Design review of the part built by this model. Coordinates are the model's own, in mm. Face numbers are marked on the shaded views. A direction names the side the tool comes from. Give positions to 0.01 mm unless a question says otherwise; leave off trailing zeros. Write each loop counter-clockwise with the first axis right and the second up, starting at its lowest first coordinate (ties: lowest second). Pieces come first, ordered by that corner, then holes.
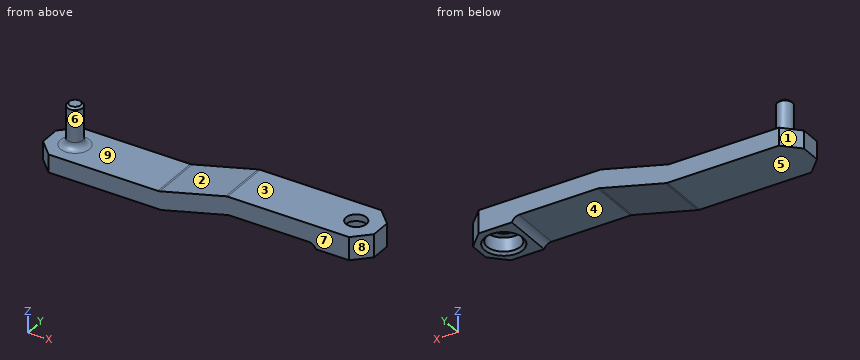
```python
from build123d import *

# Parameters (mm, degrees)
BOSS_EXTRUDE1_DEPTH = 12.7
SKETCH2_R           = 4.1148
CUT_EXTRUDE1_DEPTH  = 4.064
SKETCH3_R           = 2.54
CUT_EXTRUDE2_DEPTH  = 84.509486698
SKETCH4_R           = 1.9304
BOSS_EXTRUDE2_DEPTH = 10.16
FILLET1_R           = 1.651
CHAMFER1_SIZE       = 3.81
FILLET2_R           = 1.905
CHAMFER2_SIZE       = 0.635
CHAMFER3_SIZE       = 0.508


with BuildPart() as part:
    # Sketch1 → Boss-Extrude1 (new body)
    with BuildSketch(Plane(origin=(0, 0, 0), x_dir=(1, 0, 0), z_dir=(0, 1, 0))):
        Polygon((0, 0), (0, -4.445), (31.190740793, -4.445), (48.018240793, -8.7475), (82.2325, -8.7475), (82.2325, -3.0325), (70.1675, -3.0325), (70.1675, -4.3025), (48.5775, -4.3025), (31.75, 0), align=None)
    extrude(amount=BOSS_EXTRUDE1_DEPTH)

    # Sketch2 → Cut-Extrude1 (cut)
    with BuildSketch(Plane(origin=(0, 0, 3.0325), x_dir=(-1, 0, 0), z_dir=(0, 0, -1))):
        with Locations((-76.2, 6.35)):
            Circle(SKETCH2_R)
    extrude(amount=-CUT_EXTRUDE1_DEPTH, mode=Mode.SUBTRACT)

    # Sketch3 → Cut-Extrude2 (cut, through all)
    with BuildSketch(Plane(origin=(0, 0, 7.0965), x_dir=(-1, 0, 0), z_dir=(0, 0, -1))):
        with Locations((-76.2, 6.35)):
            Circle(SKETCH3_R)
    extrude(amount=-CUT_EXTRUDE2_DEPTH, mode=Mode.SUBTRACT)

    # Sketch4 → Boss-Extrude2 (add)
    with BuildSketch(Plane(origin=(0, 0, 4.445), x_dir=(-1, 0, 0), z_dir=(0, 0, -1))):
        with Locations((-6.35, 6.35)):
            Circle(SKETCH4_R)
    extrude(amount=-BOSS_EXTRUDE2_DEPTH)

    # Fillet1
    fillet1_edges = [part.edges().sort_by_distance(p)[0] for p in [
        (8.2804, 6.35, 4.445),
    ]]
    fillet(fillet1_edges, radius=FILLET1_R)

    # Chamfer1
    chamfer1_edges = [part.edges().sort_by_distance(p)[0] for p in [
        (82.2325, 0, 5.89),
        (0, 0, 2.2225),
        (82.2325, 12.7, 5.89),
        (0, 12.7, 2.2225),
    ]]
    chamfer(chamfer1_edges, length=CHAMFER1_SIZE)

    # Fillet2
    # the kernel refuses this fillet: 1.905 mm, written as the material it adds along each edge
    with BuildSketch(Plane(origin=(31.190740793, 0, 4.445), x_dir=(-1, 0, 0), z_dir=(0, 1, 0))) as fillet2_piece_1:
        with BuildLine():
            CenterArc((FILLET2_R * 0.125817594312, FILLET2_R), FILLET2_R, 255.657728572, 14.342271428)
            Line((-FILLET2_R * 0.121896267277, FILLET2_R * 0.0311667621428), (0, 0))
            Line((0, 0), (FILLET2_R * 0.125817594312, 0))
        make_face()
    extrude(amount=12.7)
    with BuildSketch(Plane(origin=(48.5775, 0, 4.3025), x_dir=(-0.96883323785722, 0, -0.24771386158851796), z_dir=(0, 1, 0))) as fillet2_piece_2:
        with BuildLine():
            CenterArc((FILLET2_R * 0.125817594312, -FILLET2_R), FILLET2_R, 90, 14.342271428)
            Line((-FILLET2_R * 0.121896267277, -FILLET2_R * 0.0311667621428), (0, 0))
            Line((0, 0), (FILLET2_R * 0.125817594312, 0))
        make_face()
    extrude(amount=12.7)
    with BuildSketch(Plane(origin=(70.1675, 0, 4.3025), x_dir=(-1, 0, 0), z_dir=(0, 1, 0))) as fillet2_piece_3:
        with BuildLine():
            CenterArc((1.796051224, -1.905), FILLET2_R, 90, 70.528779366)
            Line((0, -1.27), (0, 0))
            Line((0, 0), (1.796051224, 0))
        make_face()
    extrude(amount=12.7)
    # the kernel refuses this fillet: 1.905 mm, written as the material it takes off along each edge
    with BuildSketch(Plane(origin=(48.018240793, -0.599206293, 8.7475), x_dir=(-0.96883323785722, 0, -0.24771386158851796), z_dir=(0, 1, 0))) as fillet2_2_piece_1:
        with BuildLine():
            CenterArc((FILLET2_R * 0.125817594312, -FILLET2_R), FILLET2_R, 90, 14.342271428)
            Line((-FILLET2_R * 0.121896267277, -FILLET2_R * 0.0311667621428), (0, 0))
            Line((0, 0), (FILLET2_R * 0.125817594312, 0))
        make_face()
    extrude(amount=13.898412586, mode=Mode.SUBTRACT)
    with BuildSketch(Plane(origin=(31.75, -0.599206293, 0), x_dir=(-1, 0, 0), z_dir=(0, 1, 0))) as fillet2_2_piece_2:
        with BuildLine():
            CenterArc((FILLET2_R * 0.125817594312, FILLET2_R), FILLET2_R, 255.657728572, 14.342271428)
            Line((-FILLET2_R * 0.121896267277, FILLET2_R * 0.0311667621428), (0, 0))
            Line((0, 0), (FILLET2_R * 0.125817594312, 0))
        make_face()
    extrude(amount=13.898412586, mode=Mode.SUBTRACT)

    # Chamfer2
    chamfer2_edges = [part.edges().sort_by_distance(p)[0] for p in [
        (80.3148, 6.35, 3.0325),
    ]]
    chamfer(chamfer2_edges, length=CHAMFER2_SIZE)

    # Chamfer3
    chamfer3_edges = [part.edges().sort_by_distance(p)[0] for p in [
        (8.2804, 6.35, 14.605),
    ]]
    chamfer(chamfer3_edges, length=CHAMFER3_SIZE)


solid = part.part
```
(1) Mouldability with a two-part tool opening along X and no side actions: class the marked faces 6, 7, 8 and 9 as pulls with the +X half, pulls with the -X half, needs draft (parallel to the pull), parting line crosses it, or undercut.
Resolved:
face 6: undercut
face 7: needs draft
face 8: pulls with the +X half
face 9: undercut
(2) Consider section D-D, the plane z = 2. Give the boundary of the cut face in (x, y).
Resolved:
outline: (0, 3.81) - (3.81, 0) - (39.57, 0) - (39.57, 12.7) - (3.81, 12.7) - (0, 8.89) - close
(3) Tool access review of the marked faces 1, 2, 3, 4 and 5: name each direction out of +Z, -Z, +X, -X, +Y, -Y from which nothing blocks a thin tool from reaching the whole face with its end or side.
Resolved:
face 1: +Z, -Z, -X, +Y
face 2: +Z, +Y, -Y
face 3: +Z, +X, +Y, -Y
face 4: -Z, +Y, -Y
face 5: -Z, +X, -X, +Y, -Y
(4) To check wall thickness, follow L1, parallel to Y at x = 76.2, z = 7.9; L2, parallel to Z at x = 56, y = 5.5; L3, parallel to Z at x = 27.5, y = 9.25 (3 decimals). State the ranges of each line that lie inside material, in increasing order.
Resolved:
L1: y = 0 to 3.81, 8.89 to 12.7
L2: z = 4.3 to 8.75
L3: z = 0 to 4.445
(5) Consider section C-C, the plane x = 6.35. Give the boundary of the cut face in (y, z) (3 decimals).
Resolved:
outline: (0, 0) - (12.7, 0) - (12.7, 4.445) - (9.931, 4.445) arc R1.651 cw to (8.28, 6.096) - (8.28, 14.097) - (7.772, 14.605) - (4.928, 14.605) - (4.42, 14.097) - (4.42, 6.096) arc R1.651 cw to (2.769, 4.445) - (0, 4.445) - close
(6) Consider section A-A, the plane x = 76.2. Give the boundary of the cut face in (y, z), then the cut area to 3 significant figures.
Resolved:
outline: (0, 3.03) - (1.6, 3.03) - (2.24, 3.67) - (2.24, 7.1) - (3.81, 7.1) - (3.81, 8.75) - (0, 8.75) - close; (8.89, 7.1) - (10.46, 7.1) - (10.46, 3.67) - (11.1, 3.03) - (12.7, 3.03) - (12.7, 8.75) - (8.89, 8.75) - close
area: 30.3 mm2
(7) Clearance check with flat-ended pins moving along their axes: P1, Ø2, axis at x = 29.5, z = 4.5, coming from the -Y side; P2, Ø1, axis at x = 69, y = 7.5, coming from the +Z side; P3, Ø3.5, axis at x = 77, y = 5, coming from the -Z side. State where each tip first meets the part, or that it passes through.
Resolved:
P1: stops at y = 0
P2: stops at z = 8.75
P3: stops at z = 7.1
